from build123d import *

# Parameters (mm, degrees)
SKETCH1_R                                       = 13.5
SKETCH1_R_2                                     = 1.6
BOSS_EXTRUDE1_DEPTH                             = 10
SKETCH2_R                                       = 2.5
BOSS_EXTRUDE2_DEPTH                             = 35.8
SKETCH3_R                                       = 2.3
CUT_EXTRUDE1_DEPTH                              = 6
CSK_FOR_M3_FLAT_HEAD_MACHINE_SCREW1_D           = 3.4
CSK_FOR_M3_FLAT_HEAD_MACHINE_SCREW1_CSINK_D     = 6.3
CSK_FOR_M3_FLAT_HEAD_MACHINE_SCREW1_CSINK_ANGLE = 90


with BuildPart() as part:
    # Sketch1 → Boss-Extrude1 (new body)
    with BuildSketch(Plane.XY):
        Circle(SKETCH1_R)
        with Locations((0, 9)):
            Circle(SKETCH1_R_2, mode=Mode.SUBTRACT)
        with Locations((0, -9)):
            Circle(SKETCH1_R_2, mode=Mode.SUBTRACT)
        with Locations((-9, 0)):
            Circle(SKETCH1_R_2, mode=Mode.SUBTRACT)
        with Locations((9, 0)):
            Circle(SKETCH1_R_2, mode=Mode.SUBTRACT)
    extrude(amount=BOSS_EXTRUDE1_DEPTH)

    # Sketch2 → Boss-Extrude2 (add)
    with BuildSketch(Plane.XY.offset(10)):
        with Locations(Location((0, 0, 0), (0, 0, 180))):
            Circle(SKETCH2_R)
    extrude(amount=BOSS_EXTRUDE2_DEPTH)

    # Sketch3 → Cut-Extrude1 (cut)
    with BuildSketch(Plane(origin=(0, 0, 0), x_dir=(-1, 0, 0), z_dir=(0, 0, -1))):
        Circle(SKETCH3_R)
    extrude(amount=-CUT_EXTRUDE1_DEPTH, mode=Mode.SUBTRACT)

    # CSK for M3 Flat Head Machine Screw1 (through all)
    with Locations(Plane.XY.offset(10)):
        with Locations((0, 9), (9, 0), (-9, 0), (0, -9)):
            CounterSinkHole(CSK_FOR_M3_FLAT_HEAD_MACHINE_SCREW1_D / 2, CSK_FOR_M3_FLAT_HEAD_MACHINE_SCREW1_CSINK_D / 2, counter_sink_angle=CSK_FOR_M3_FLAT_HEAD_MACHINE_SCREW1_CSINK_ANGLE)


solid = part.part
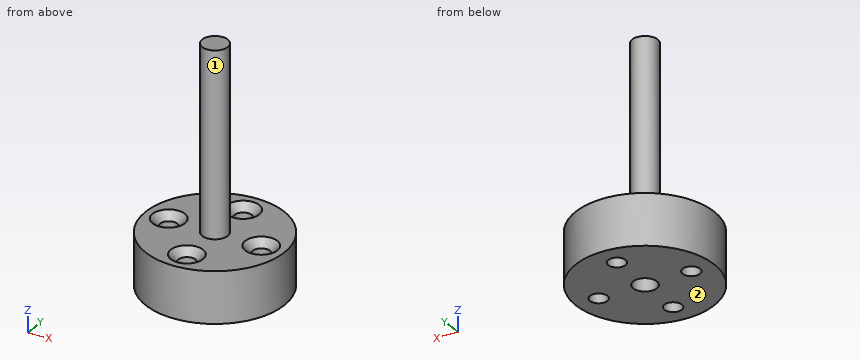
Could you check a few things on this model? Use its own coordinates, in mm. Face numbers are marked on the shaded views. A direction names the side the tool comes from. Round coordinates to 2 decimals unless told otherwise and drop trailing zeros. Order: outer loops, then holes, each group sorted by start corner. A loop starts at its lowest first (then second) coordinate and runs counter-clockwise, first axis right, second up.
Q1. Which directions (+Z, -Z, +X, -X, +Y, -Y) give clear straight access to the entire face, cutting with the end or side of a thin tool? Please do the marked faces 1 and 2.
Geometry says:
face 1: +Z
face 2: -Z, +X, -X, +Y, -Y
Q2. Imagine slicing it at D-D, the plane z = 8. List the corners of the cut face in (x, y) for me.
Geometry says:
outline: circle Ø27 at (0, 0); hole circle Ø3.4 at (-9, 0); hole circle Ø3.4 at (0, -9); hole circle Ø3.4 at (0, 9); hole circle Ø3.4 at (9, 0)
Q3. Please list where these lines run through material, in increasing order: probe 1 along Y at (x, z) = (0, 3); probe 2 along Z at (x, y) = (11.75, 6); probe 3 along Y at (x, z) = (-9, 2.25).
Geometry says:
probe 1: y = -13.5 to -10.7, -7.3 to -2.3, 2.3 to 7.3, 10.7 to 13.5
probe 2: z = 0 to 10
probe 3: y = -10.06 to -1.7, 1.7 to 10.06
Q4. Imagine slicing it at A-A, the plane y = 0. List the corners of the cut face in (x, z) for me.
Geometry says:
outline: (-13.5, 0) - (-10.7, 0) - (-10.7, 8.55) - (-12.15, 10) - (-13.5, 10) - close; (-7.3, 0) - (-2.3, 0) - (-2.3, 6) - (2.3, 6) - (2.3, 0) - (7.3, 0) - (7.3, 8.55) - (5.85, 10) - (2.5, 10) - (2.5, 45.8) - (-2.5, 45.8) - (-2.5, 10) - (-5.85, 10) - (-7.3, 8.55) - close; (10.7, 0) - (13.5, 0) - (13.5, 10) - (12.15, 10) - (10.7, 8.55) - close
Q5. I'm going to push flat-ended pins straight in: P1, Ø4, axis at x = 9, y = 0, coming from the +Z side; P2, Ø1, axis at x = -5, y = 8, coming from the +Z side; P3, Ø2.5, axis at x = 0, y = 9, coming from the -Z side; P4, Ø1.5, axis at x = 7, z = 9.5, coming from the +Y side. Where does each tip first touch, or does it pass through?
Geometry says:
P1: stops at z = 8.85
P2: stops at z = 10
P3: passes through
P4: stops at y = 11.97
Q6. Imagine slicing it at B-B, the plane z = 3. List the corners of the cut face in (x, y) for me, then the cut area to 3 significant figures.
Geometry says:
outline: circle Ø27 at (0, 0); hole circle Ø3.4 at (-9, 0); hole circle Ø4.6 at (0, 0); hole circle Ø3.4 at (0, -9); hole circle Ø3.4 at (0, 9); hole circle Ø3.4 at (9, 0)
area: 520 mm2
